from build123d import *

# Parameters (mm, degrees)
F0_W     = 508
F0_H     = 508
F1_DEPTH = 508
F3_D     = 152.4
F4_T     = -2.54


with BuildPart() as f1:
    # F0 (on Top) → F1 (new body)
    with BuildSketch(Plane.XY):
        Rectangle(F0_W, F0_H)
    extrude(amount=F1_DEPTH)

    # F3 (through all)
    with Locations(Plane.XZ.offset(254)):
        with Locations((0, 254)):
            Hole(F3_D / 2)

    # F4 (hollow: no face is removed)
    offset(amount=F4_T, mode=Mode.SUBTRACT)


solid = f1.part
Model file for the job. Use its own axes, mm. A direction names the side the tool comes from. Round coordinates to 2 decimals unless told otherwise and drop trailing zeros. Loops run counter-clockwise (first coordinate to the right, second up) from the corner with the lowest first, then second, coordinate; pieces in that order, holes last.
1. Band-saw the part on B-B, the plane z = 254. List the corners of the cut face in (x, y).
Check values:
outline: (-254, -254) - (-76.2, -254) - (-76.2, 254) - (-254, 254) - close; (76.2, -254) - (254, -254) - (254, 254) - (76.2, 254) - close; hole (-251.46, -251.46) - (-78.74, -251.46) - (-78.74, 251.46) - (-251.46, 251.46) - close; hole (78.74, -251.46) - (251.46, -251.46) - (251.46, 251.46) - (78.74, 251.46) - close
2. Wall check: probe 1 along Z at (x, y) = (0, 76.5); probe 2 along Z at (x, y) = (4.5, 167); probe 3 along Y at (x, z) = (167.5, 57.5). Give the ranges that are in metal, low to high.
Check values:
probe 1: z = 0 to 2.54, 175.26 to 177.8, 330.2 to 332.74, 505.46 to 508
probe 2: z = 0 to 2.54, 175.39 to 177.93, 330.07 to 332.61, 505.46 to 508
probe 3: y = -254 to -251.46, 251.46 to 254
3. Mould opens along Z. For faces 3 (the flat face through (-4, 4, 508)), 4 (the flat face through (-4, 4, 0)), 5 (the flat face through (-4, 4, 505.46)) say: +Z half, -Z half, draft (parallel to the pull), parting line (faces both ways), or undercut.
Check values:
face 3: +Z half
face 4: -Z half
face 5: undercut
4. Tool access for faces 1 (the flat face through (-59, 251.46, 195)), 2 (the flat face through (-254, -4, 250)): list every direction of +Z, -Z, +X, -X, +Y, -Y with a clear straight run to the whole face (end or side of a thin tool).
Check values:
face 1: none
face 2: +Z, -Z, -X, +Y, -Y
5. Band-saw the part on D-D, the plane x = -169. List the corners of the cut face in (y, z).
Check values:
outline: (-254, 0) - (254, 0) - (254, 508) - (-254, 508) - close; hole (-251.46, 2.54) - (251.46, 2.54) - (251.46, 505.46) - (-251.46, 505.46) - close
6. Band-saw the part on A-A, the plane x = 0. List the corners of the cut face in (y, z).
Check values:
outline: (-254, 0) - (254, 0) - (254, 177.8) - (-254, 177.8) - close; (-254, 330.2) - (254, 330.2) - (254, 508) - (-254, 508) - close; hole (-251.46, 2.54) - (251.46, 2.54) - (251.46, 175.26) - (-251.46, 175.26) - close; hole (-251.46, 332.74) - (251.46, 332.74) - (251.46, 505.46) - (-251.46, 505.46) - close
7. Band-saw the part on C-C, the plane y = 152.5. List the corners of the cut face in (x, z).
Check values:
outline: (-254, 0) - (254, 0) - (254, 508) - (-254, 508) - close; circle Ø157.48 at (0, 254); hole (-251.46, 2.54) - (251.46, 2.54) - (251.46, 505.46) - (-251.46, 505.46) - close; hole circle Ø152.4 at (0, 254)
